Geometry: final body of the model. Coordinates: model frame, mm. A direction names the side the tool comes from. Round coordinates to 2 decimals unless told otherwise and drop trailing zeros. Put each result on its own line as item: value. Start each with the question number.
(1) Material intervals for L1, parallel to Z at x = 41.5, y = -6.25; L2, parallel to Y at x = -42.5, z = 15; L3, parallel to X at y = 8.75, z = -4, sorted ascending. Write a range as [from, to].
(2) Pin query (flat end, axial travel): P1, Ø5, axis at y = -4.5, z = -3.5, coming from the -X side; P2, Ø11.5, axis at x = -2.5, y = 3, coming from the +Z side; P3, Ø2, axis at x = 17.5, y = 6.5, coming from the -Z side. Return the tip coordinate at first contact, or that it passes through.
(3) Access query for faces 1 (the face through (-42.3, 3.4, -19.3)), 2 (the face through (14, 0, -16.8)), 3 (the face through (-32, 0, 16.8)), 4 (the face through (-46.3, 1.4, 18.3)). Directions: +Z, -Z, +X, -X, +Y, -Y. A direction counts if a zero-diameter tool reaches every point of the face in a straight line with its end or side. Return the directions, or none.
from build123d import *

# Parameters (mm, degrees)
SKETCH1_W           = 104.4
SKETCH1_H           = 33.6
BOSS_EXTRUDE1_DEPTH = 12.7
FILLET1_R           = 10
SKETCH2_R           = 1.9
BOSS_EXTRUDE2_DEPTH = 5
SKETCH4_R           = 0.95
BOSS_EXTRUDE3_DEPTH = 3
SKETCH5_W           = 20
SKETCH5_H           = 25.4
BOSS_EXTRUDE4_DEPTH = 0.0001
BOSS_EXTRUDE5_DEPTH = 0.0001
BOSS_EXTRUDE6_DEPTH = 0.0001
FILLET7_R           = 1
FILLET8_R           = 1


with BuildPart() as part:
    # Sketch1 → Boss-Extrude1 (new body, symmetric)
    with BuildSketch(Plane(origin=(0, 0, 0), x_dir=(1, 0, 0), z_dir=(0, 1, 0))):
        Rectangle(SKETCH1_W, SKETCH1_H)
    extrude(amount=BOSS_EXTRUDE1_DEPTH, both=True)

    # Fillet1
    fillet1_edges = [part.edges().sort_by_distance(p)[0] for p in [
        (-52.2, 12.7, 0),
        (-52.2, -12.7, 0),
    ]]
    fillet(fillet1_edges, radius=FILLET1_R)

    # Sketch2 → Boss-Extrude2 (add)
    with BuildSketch(Plane(origin=(0, 0, -16.8), x_dir=(-1, 0, 0), z_dir=(0, 0, -1))):
        with Locations((44.2, 3.35)):
            Circle(SKETCH2_R)
        with Locations((44.2, -3.35)):
            Circle(SKETCH2_R)
    extrude(amount=BOSS_EXTRUDE2_DEPTH)

    # Sketch4 → Boss-Extrude3 (add)
    with BuildSketch(Plane.XY.offset(16.8)):
        with Locations((-47.2, 3.3)):
            Circle(SKETCH4_R)
        with Locations((-47.2, 1.1)):
            Circle(SKETCH4_R)
        with Locations((-47.2, -1.1)):
            Circle(SKETCH4_R)
        with Locations((-47.2, -3.3)):
            Circle(SKETCH4_R)
    extrude(amount=BOSS_EXTRUDE3_DEPTH)

    # Sketch5 → Boss-Extrude4 (add)
    with BuildSketch(Plane.XY.offset(16.8)):
        with Locations((-32.2, 0)):
            Rectangle(SKETCH5_W, SKETCH5_H)
    boss_extrude4 = extrude(amount=BOSS_EXTRUDE4_DEPTH)

    # Mirror1: Boss-Extrude4 across plane
    add(boss_extrude4.mirror(Plane.XY))

    # Mirror1 at the second plane: Boss-Extrude4 across plane
    add(boss_extrude4.mirror(Plane.ZX))

    # Sketch6 → Boss-Extrude5 (add)
    with BuildSketch(Plane(origin=(0, 12.7, 0), x_dir=(1, 0, 0), z_dir=(0, 1, 0))):
        with BuildLine():
            Line((-35.3, 13.2), (40.5, 13.2))
            ThreePointArc((40.5, 13.2), (41.914213562, 12.614213562), (42.5, 11.2))
            Line((42.5, 11.2), (42.5, -11.2))
            ThreePointArc((42.5, -11.2), (41.914213562, -12.614213562), (40.5, -13.2))
            Line((40.5, -13.2), (-35.3, -13.2))
            ThreePointArc((-35.3, -13.2), (-36.714213562, -12.614213562), (-37.3, -11.2))
            Line((-37.3, -11.2), (-37.3, 11.2))
            ThreePointArc((-37.3, 11.2), (-36.714213562, 12.614213562), (-35.3, 13.2))
        make_face()
    extrude(amount=BOSS_EXTRUDE5_DEPTH)

    # Sketch7 → Boss-Extrude6 (add)
    with BuildSketch(Plane.XZ.offset(12.7)):
        with BuildLine():
            Line((-23.4, 12.5), (27.5, 12.5))
            ThreePointArc((27.5, 12.5), (28.914213562, 11.914213562), (29.5, 10.5))
            Line((29.5, 10.5), (29.5, -10.5))
            ThreePointArc((29.5, -10.5), (28.914213562, -11.914213562), (27.5, -12.5))
            Line((27.5, -12.5), (-23.4, -12.5))
            ThreePointArc((-23.4, -12.5), (-24.814213562, -11.914213562), (-25.4, -10.5))
            Line((-25.4, -10.5), (-25.4, 10.5))
            ThreePointArc((-25.4, 10.5), (-24.814213562, 11.914213562), (-23.4, 12.5))
        make_face()
    extrude(amount=BOSS_EXTRUDE6_DEPTH)

    # Fillet7
    fillet7_edges = [part.edges().sort_by_distance(p)[0] for p in [
        (52.2, 12.7, 0),
        (-52.2, 0, 16.8),
        (-52.2, 0, -16.8),
        (15, 12.7, -16.8),
        (-49.271067812, 9.771067812, 16.8),
        (-49.271067812, -9.771067812, 16.8),
        (-49.271067812, 9.771067812, -16.8),
        (-49.271067812, -9.771067812, -16.8),
        (15, -12.7, -16.8),
        (52.2, -12.7, 0),
        (15, -12.7, 16.8),
        (15, 12.7, 16.8),
        (52.2, 0, -16.8),
        (52.2, 0, 16.8),
    ]]
    fillet(fillet7_edges, radius=FILLET7_R)

    # Fillet8
    fillet8_edges = [part.edges().sort_by_distance(p)[0] for p in [
        (-32.2, -12.7, 16.8001),
        (-32.2, 12.7, 16.8001),
        (-32.2, 12.7, -16.8001),
        (-32.2, -12.7, -16.8001),
    ]]
    fillet(fillet8_edges, radius=FILLET8_R)


solid = part.part
Checks:
1. L1: z = [-16.8, 16.8]
1. L2: y = [-12.7, 12.7]
1. L3: x = [-50.16, 52.2]
2. P1: stops at x = -52.2
2. P2: stops at z = 16.8
2. P3: stops at z = -16.8
3. face 1: -Z
3. face 2: -Z, +X, +Y, -Y
3. face 3: +Z, +X, +Y, -Y
3. face 4: +Z
